from build123d import *

# Parameters (mm, degrees)
F0_W     = 635
F0_H     = 810
F1_DEPTH = 18
F2_W     = 18
F2_H     = 30
F3_DEPTH = 623


with BuildPart() as f1:
    # F0 (on Front) → F1 (new body)
    with BuildSketch(Plane.XZ):
        Rectangle(F0_W, F0_H)
    extrude(amount=F1_DEPTH)

    # F2 (on face) → F3 (cut)
    with BuildSketch(Plane.YZ.offset(317.5)):
        with Locations((-9, 0)):
            Rectangle(F2_W, F2_H)
    extrude(amount=-F3_DEPTH, mode=Mode.SUBTRACT)


solid = f1.part
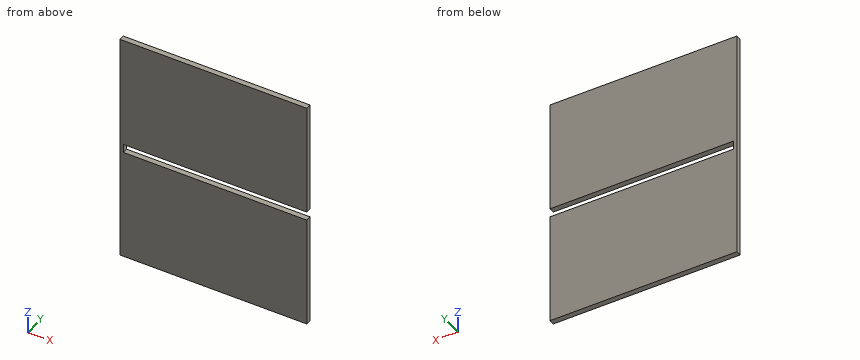
Model file for the job. Use its own axes, mm. Give positions to 0.01 mm unless a question says otherwise; leave off trailing zeros. Order: outer loops, then holes, each group sorted by start corner. A loop starts at its lowest first (then second) coordinate and runs counter-clockwise, first axis right, second up. Notation, with made-up numbers: M 56,67.5 L 105,67.5 A6 cw 105,72.5 Z; hole C 84,-9 d2. An arc over 180 degrees is marked long. Put each result on its own line as item: value. Start each with the question number.
(1) Drill centre lines: L1, parallel to Z at x = -225.5, y = -12.75; L2, parallel to X at y = -17, z = -3.5. Where is each one in solid material? Low to high. Write a range as [from, to].
(2) Pin check, flat tip, straight feed: pin 1 Ø9 at (y, z) = (-6, 6.5) entering from +X. Stop position of the tip, or through.
(3) Band-saw the part on A-A on x = -67.5. Give the cut face in (y, z).
(4) Band-saw the part on B-B on y = -10.75. Give the cut face in (x, z).
Results below:
1. L1: z = [-405, -15], [15, 405]
1. L2: x = [-317.5, -305.5]
2. pin 1: stops at x = -305.5
3. outline: M -18,-405 L 0,-405 L 0,-15 L -18,-15 Z; M -18,15 L 0,15 L 0,405 L -18,405 Z
4. outline: M -317.5,-405 L 317.5,-405 L 317.5,-15 L -305.5,-15 L -305.5,15 L 317.5,15 L 317.5,405 L -317.5,405 Z
